Autodesk Inventor part; units mm, degrees
ref_plane "Work Plane2" through (2.032, 0, 0) normal (0, 1, 0) x (1, 0, 0)
ref_plane "YZ Plane" through (0, 0, 0) normal (1, 0, 0) x (0, 1, 0)
ref_plane "XZ Plane" through (0, 0, 0) normal (0, 1, 0) x (-1, 0, 0)
sketch "Sketch1" plane through (0, 0, 0) normal (0, 0, 1) x (1, 0, 0)
  line L0 (2.1844, 0) -> (25.4, 0)
  line L1 (25.4, 0) -> (25.4, 1.7526)
  line L2 (25.4, 1.7526) -> (1.524, 1.7526)
  line L3 (0.4583, 3.0226) -> (0, 3.0226)
  line L4 (-5.08, 0) -> (30.48, 0)
  line L5 (0, -0.6045) -> (0, 3.6271)
  line L6 (0, 1.9558) -> (1.5573, 1.1793)
  line L7 (1.5573, 1.1793) -> (2.1844, 0)
  line L8 (1.524, 1.7526) -> (0.4583, 3.0226)
  line L9 (0, 3.0226) -> (0, 1.9558)
  dimension "d2" = 3.5052
  dimension "d3" = 6.0452
  dimension "d4" = 2.1844
  dimension "d5" = 3.9116
  dimension "d6" = 26.5
  dimension "d7" = 62
  dimension "d13" = 50
  dimension "d14" = 1.524
  dimension "d15" = 25.4
revolve "Body" add sketch "Sketch1" angle 360 about axis through (2.1844, 0, 0) along (1, 0, 0) contours L7 L6 L5 L3 L8 L2 L1 L0
sketch "Sketch2" plane through (0, 0, 0) normal (-1, 0, 0) x (0, 0, 1)
  line L0 (0, -4.2316) -> (0, 4.2316)
  line L1 (-4.2316, 0) -> (4.2316, 0)
  line L2 (0, 1.9558) -> (0, 0) construction
  line L3 (0, 0) -> (1.9558, 0) construction
  arc A0 (0.6519, 0) -> (0, 0.6519) centre (0, 0) ccw
  line L4 (0, 0) -> (0.7947, 0.7947) construction
  arc A1 (0.9779, 0) -> (0, 0.9779) centre (0, 0) ccw construction
  line L5 (0.3429, 1.9255) -> (0.2811, 0.9366)
  line L6 (1.9255, 0.3429) -> (0.9366, 0.2811)
  arc A2 (0.2811, 0.9366) -> (0.9366, 0.2811) centre (0.8981, 0.8981) ccw
  arc A3 (1.9558, 0) -> (1.9255, 0.3429) centre (0, 0) ccw
  arc A4 (0.3429, 1.9255) -> (0, 1.9558) centre (0, 0) ccw
  arc A5 (1.9255, 0.3429) -> (0.3429, 1.9255) centre (0, 0) ccw
  line L7 (0.3429, -1.9255) -> (0.2811, -0.9366)
  line L8 (1.9255, -0.3429) -> (0.9366, -0.2811)
  arc A6 (0.9366, -0.2811) -> (0.2811, -0.9366) centre (0.8981, -0.8981) ccw
  arc A7 (1.9255, -0.3429) -> (1.9558, 0) centre (0, 0) ccw
  arc A8 (0, -1.9558) -> (0.3429, -1.9255) centre (0, 0) ccw
  arc A9 (0.3429, -1.9255) -> (1.9255, -0.3429) centre (0, 0) ccw
  line L9 (-0.3429, 1.9255) -> (-0.2811, 0.9366)
  line L10 (-1.9255, 0.3429) -> (-0.9366, 0.2811)
  arc A10 (-0.9366, 0.2811) -> (-0.2811, 0.9366) centre (-0.8981, 0.8981) ccw
  arc A11 (-1.9255, 0.3429) -> (-1.9558, 0) centre (0, 0) ccw
  arc A12 (0, 1.9558) -> (-0.3429, 1.9255) centre (0, 0) ccw
  arc A13 (-0.3429, 1.9255) -> (-1.9255, 0.3429) centre (0, 0) ccw
  arc A14 (-1.9255, -0.3429) -> (-0.3429, -1.9255) centre (0, 0) ccw
  arc A15 (-0.3429, -1.9255) -> (0, -1.9558) centre (0, 0) ccw
  arc A16 (-1.9558, 0) -> (-1.9255, -0.3429) centre (0, 0) ccw
  line L11 (-1.9255, -0.3429) -> (-0.9366, -0.2811)
  arc A17 (-0.2811, -0.9366) -> (-0.9366, -0.2811) centre (-0.8981, -0.8981) ccw
  line L12 (-0.3429, -1.9255) -> (-0.2811, -0.9366)
  dimension "d18" = 45
  dimension "d19" = 1.3039
  dimension "d20" = 1.9558
  dimension "d21" = 3.9116
  dimension "d22" = 0.3429
extrude "Slot" add sketch "Sketch2" against normal up to next contours A2 L5 A5 L6 | L9 A10 L10 A13 | L7 A6 L8 A9 | A14 L11 A17 L12
fillet "Fillet1" radius 0.1372 4 edges at (0, 1.9558, 0) (0, 0, 1.9558) (0, -1.9558, 0) (0, 0, -1.9558)
thread "Thread"
chamfer "Chamfer1" distance 0.4723 distance2 0.4723 1 edges at (25.4, -1.7526, 0) measured on face at (25.4, -0.4373, -0.5742)
ref_plane "Work Plane2" through (2.032, 0, 0) normal (0, 1, 0) x (1, 0, 0)
equation "\"d2\" = GD"
equation "\"d3\" = KOD"
equation "\"d4\" = INTI"
equation "\"d5\" = SDM"
equation "\"d13\" = 0.5 * SEWI"
equation "\"d14\" = KOH"
equation "\"d15\" = NLG"
equation "\"d19\" = 0.333333 * SDM"
equation "\"d20\" = 0.5 * SDM"
equation "\"d21\" = SDM"
equation "\"d22\" = 0.5 * SBR"
equation "\"d45\" = INTI"
equation "\"d25\" = 0.2 * SBR"
equation "\"d9\" = GEL"
equation "\"d11\" = -0.5 * SPD + 0.5 * GD"
equation "\"d12\" = GUL"
equation "\"GD\" = NND"
equation "\"NLG\" = 25.4"
equation "\"GEL\" = 19.05"
equation "\"KOD\" = 6.0452"
equation "\"KOH\" = 1.524"
equation "\"SDM\" = 3.9116"
equation "\"INTI\" = 2.1844"
equation "\"SBR\" = 0.6858"
equation "\"GUL\" = -0.5 * SPD + 0.5 * NND"
equation "\"SPD\" = 2.56064"
equation "\"SEWI\" = 100deg"
equation "\"d0\" = NLG"
equation "\"d1\" = KOH"
equation "\"d17\" = SDM"
equation "\"TOA\" = 30deg"
equation "\"EPV\" = 2.99461"
equation "\"THREADDIA\" = 3.5052"
equation "\"BDM\" = NND"
equation "\"NND\" = 3.5052"
equation "\"GAL\" = 0.79375"
equation "\"GD1\" = SPD"
properties part number "ANSI B18.6.3 - 6-32 UNC x 1, CRFCHMSTII(2)" material "Steel, Mild"
The listing builds one solid part. Answer for the finished solid, in the listing's coordinates (mm). A direction names the side the tool comes from. Coordinates: 2 decimals unless noted, no trailing zeros. Order: outer loops, then holes, each group sorted by start corner. A loop starts at its lowest first (then second) coordinate and runs counter-clockwise, first axis right, second up.
Q1. Consider line 1 (Z direction, x = 13.5, y = 0); line 2 (Z direction, x = 1.75, y = 0.5); line 3 (Z direction, x = 19.25, y = -1). Determine where each line is inside the solid, lowest interval first.
Q2. Given P1, Ø3, axis at x = 4, y = -0.5, coming from the -Z side; P2, Ø1.5, axis at x = 8.5, z = -1.5, coming from the +Y side; P3, Ø1.5, axis at x = 2.5, y = 1.5, coming from the -Z side, each flat-ended and moving along its own axis, determine where each tip first touches the part or whether it passes through.
Q3. Which of the six approach directions +Z, -Z, +X, -X, +Y, -Y give full straight-line access (tool end or side, diameter ignored) to faces 4 (the face through (0, 1, -1)), 5 (the face through (0.64, 0.3, -1.24))?
Q4. For a pull along Y with two mould halves and no side action, classify faces 1 (the face through (0.64, -1.24, 0.3)), 2 (the face through (13.06, 1.67, -0.53)), 3 (the face through (25.4, 0, 0)) as pulls with the +Y half, pulls with the -Y half, needs draft (parallel to the pull), parting line crosses it, or undercut.
Q5. A cutting plane is placed at A-A, the plane x = 6. Write down the section's boundary in (y, z), and give its area (3 significant figures).
Answers follow:
1. line 1: z = -1.75 to 1.75
1. line 2: z = -1.68 to -0.43, 0.43 to 1.68
1. line 3: z = -1.44 to 1.44
2. P1: stops at z = -1.75
2. P2: stops at y = 1.58
2. P3: stops at z = -1.58
3. face 4: +Z, -Z, -X, +Y, -Y
3. face 5: -X
4. face 1: undercut
4. face 2: parting line crosses it
4. face 3: needs draft
5. outline: circle Ø3.51 at (0, 0)
5. area: 9.65 mm2
